Drawing for the job (mm, zero at the part's lowest x, y, z). A direction names the side the tool comes from. Round coordinates to 2 decimals unless told otherwise and drop trailing zeros. Write each loop counter-clockwise with the first axis right and the second up, starting at its lowest first coordinate (ties: lowest second). Pieces come first, ordered by that corner, then holes. Notation, with made-up numbers: (11.25, 37) -> (64.25, 37) arc R28 ccw to (64.25, 69) -> close; hole circle Ø11 at (-17, 35.5). An arc over 180 degrees is marked (long way). Answer in a Markdown table with one row per item. Add a question column.
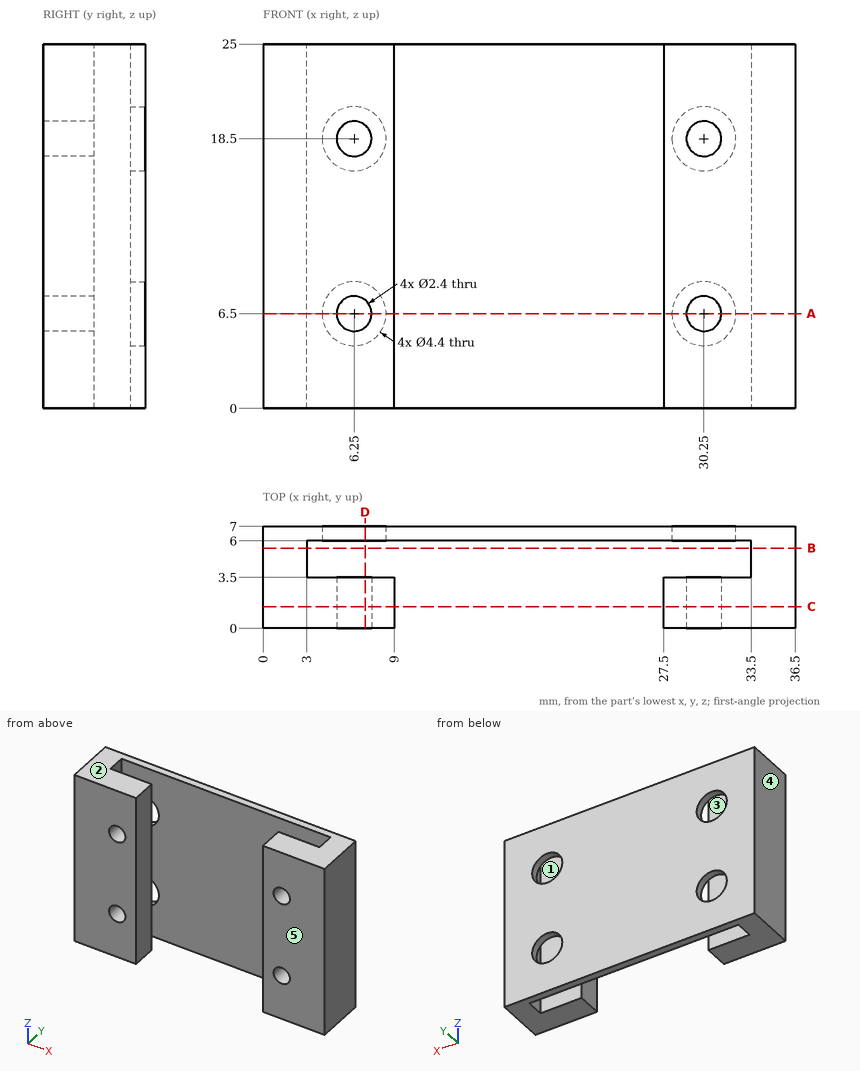
(1) Probe line 1 along Z through (x, y) = (6.25, 6.3); line 2 along X through (y, z) = (2.4, 18.5); line 3 along Z through (x, y) = (30.25, 2.3). List the from-to ranges inside material, lowest first.
(2) Saw through at D-D (x = 7). List the corners of the cut face in (y, z), plus the area to 3 significant figures.
(3) Drop flat-ended pins along their axis: P1, Ø3, axis at x = 6.25, z = 6.5, coming from the -Y side; P2, Ø2.5, axis at x = 6.25, z = 6.5, coming from the +Y side. Give the stop position or say it passes through.
(4) Saw through at C-C (y = 1.5). List the corners of the cut face in (x, z).
(5) Saw through at B-B (y = 5.5). List the corners of the cut face in (x, z), plus the area to 3 significant figures.
(6) Mould opens along X. For the marked faces 3, 4 and 5 say: pulls with the +X half, pulls with the -X half, needs draft (parallel to the pull), parting line crosses it, or undercut.
(7) Saw through at A-A (z = 6.5). List the corners of the cut face in (x, y), plus the area to 3 significant figures.
(8) Which spindle directions (+Z, -Z, +X, -X, +Y, -Y) get a long thin tool onto all of the face, cutting with end or side? Do the marked faces 1 and 2. Say none if no direction does.
Answer sheet:
| question | item | result |
|---|---|---|
| 1 | line 1 | z = 0 to 4.3, 8.7 to 16.3, 20.7 to 25 |
| 1 | line 2 | x = 0 to 5.05, 7.45 to 9, 27.5 to 29.05, 31.45 to 36.5 |
| 1 | line 3 | z = 0 to 5.3, 7.7 to 17.3, 19.7 to 25 |
| 2 | outline | (0, 0) -> (3.5, 0) -> (3.5, 5.56) -> (0, 5.56) -> close; (0, 7.44) -> (3.5, 7.44) -> (3.5, 17.56) -> (0, 17.56) -> close; (0, 19.44) -> (3.5, 19.44) -> (3.5, 25) -> (0, 25) -> close; (6, 0) -> (7, 0) -> (7, 4.43) -> (6, 4.43) -> close; (6, 8.57) -> (7, 8.57) -> (7, 16.43) -> (6, 16.43) -> close; (6, 20.57) -> (7, 20.57) -> (7, 25) -> (6, 25) -> close |
| 2 | area | 91.1 mm² |
| 3 | P1 | stops at y = 0 |
| 3 | P2 | stops at y = 3.5 |
| 4 | outline | (0, 0) -> (9, 0) -> (9, 25) -> (0, 25) -> close; (27.5, 0) -> (36.5, 0) -> (36.5, 25) -> (27.5, 25) -> close; hole circle Ø2.4 at (6.25, 6.5); hole circle Ø2.4 at (6.25, 18.5); hole circle Ø2.4 at (30.25, 6.5); hole circle Ø2.4 at (30.25, 18.5) |
| 5 | outline | (0, 0) -> (3, 0) -> (3, 25) -> (0, 25) -> close; (33.5, 0) -> (36.5, 0) -> (36.5, 25) -> (33.5, 25) -> close |
| 5 | area | 150 mm² |
| 6 | face 3 | undercut |
| 6 | face 4 | pulls with the -X half |
| 6 | face 5 | needs draft |
| 7 | outline | (0, 0) -> (5.05, 0) -> (5.05, 3.5) -> (3, 3.5) -> (3, 6) -> (4.05, 6) -> (4.05, 7) -> (0, 7) -> close; (7.45, 0) -> (9, 0) -> (9, 3.5) -> (7.45, 3.5) -> close; (8.45, 6) -> (28.05, 6) -> (28.05, 7) -> (8.45, 7) -> close; (27.5, 0) -> (29.05, 0) -> (29.05, 3.5) -> (27.5, 3.5) -> close; (31.45, 0) -> (36.5, 0) -> (36.5, 7) -> (32.45, 7) -> (32.45, 6) -> (33.5, 6) -> (33.5, 3.5) -> (31.45, 3.5) -> close |
| 7 | area | 88.9 mm² |
| 8 | face 1 | +Z, -Z |
| 8 | face 2 | +Z, +X, -X, +Y, -Y |
